Design review of the part built by this model. Coordinates are the model's own, in mm. A direction names the side the tool comes from. Round coordinates to 2 decimals unless told otherwise and drop trailing zeros. Loops run counter-clockwise (first coordinate to the right, second up) from the corner with the lowest first, then second, coordinate; pieces in that order, holes last. Notation, with made-up numbers: (8.25, 56) -> (47.25, 56) arc R6 ccw to (47.25, 63) -> close; hole circle Ø8 at (30, -37). An arc over 180 degrees is marked (long way). Answer as CSV lines item,"result". Start each with the question number.
(1) For P1, Ø1.5, axis at y = -10, z = 22, coming from the +X side; P2, Ø8.5, axis at x = -106, y = -23, coming from the +Z side; P3, Ø9.5, axis at x = -102.5, y = -17, coming from the -Z side, all flat-tipped, find the tip position at first contact; note any pin that passes through.
(2) To check wall thickness, follow line 1 (X direction, y = -15, z = 33); line 2 (Y direction, x = -36.5, z = 17); line 3 (X direction, y = -8.5, z = 16). State the ranges of each line that lie inside material, in increasing order. Write a range as from..to.
(3) Draft analysis for pull direction X (two halves, no side actions). For faces 4 (the face through (115.983, -17.769, -24.608)), 5 (the face through (-115.983, -17.769, -24.608)), 6 (the face through (114.96, -17.69, 11.75)), state which applies: +X half, -X half, draft (parallel to the pull), parting line (faces both ways), or undercut.
(4) Take a section at B-B, the plane y = -23. Write out the cut boundary in (x, z), and give its area (3 significant figures).
(5) Take a section at C-C, the plane x = 66. Write out the cut boundary in (y, z), and give its area (3 significant figures).
(6) Machinability: for faces 1 (the face through (-1, -2, 48.064)), 2 (the face through (100, -19, -33.216)), 3 (the face through (101, -19, -25.596)), which of the approach directions +Z, -Z, +X, -X, +Y, -Y give a long, thin tool a straight path to every point of the face, cutting with its end or side? Answer none if there is none.
(7) Take a section at D-D, the plane z = -22. Write out the cut boundary in (x, y), and give its area (3 significant figures).
(8) Take a section at A-A, the plane z = -8. Write out the cut boundary in (x, y), and give its area (3 significant figures).
from build123d import *

# Parameters (mm, degrees)
F0_W     = 246.3848441839
F0_H     = 96.1289182305
F1_DEPTH = 3.81
F2_R     = 14.1092662394
F3_DEPTH = 81.28
F5_DEPTH = 25.4
F6_R     = 14.1092662394
F7_DEPTH = 7.62


# Not quite as in the source:
# - a pattern or mirror of a feature is missing from the dataset's text; its kind, count and spacing are read off the source's solid
# - a feature names something its author has since deleted; it is built from what else it names


with BuildPart() as f1:
    # F0 (on Front) → F1 (new body)
    with BuildSketch(Plane.XZ):
        Rectangle(F0_W, F0_H)
    extrude(amount=F1_DEPTH)

    # F2 (on face) → F3 (join)
    with BuildSketch(Plane.XY.offset(48.0644591153)):
        with BuildLine():
            ThreePointArc((-108.1859269769, -3.81), (-109.4788428986, -32.8031453268), (-84.1323126967, -18.6671093106))
            ThreePointArc((-84.1323126967, -18.6671093106), (-86.6114524229, -9.9357548511), (-93.3090499012, -3.81))
            Line((-93.3090499012, -3.81), (-108.1859269769, -3.81))
        make_face()
        with Locations((-100.8657291532, -18.3125622571)):
            Circle(F2_R, mode=Mode.SUBTRACT)
    f3 = extrude(amount=-F3_DEPTH)

    # F3_copies: F3 across plane
    add(f3.mirror(Plane(origin=(0, 0, 0), x_dir=(0, 0, 1), z_dir=(1, 0, 0))))

    # F4 (on face) → F5 (cut)
    with BuildSketch(Plane(origin=(0, 0, 0), x_dir=(-1, 0, 0), z_dir=(0, 1, 0))):
        Polygon((-113.6597358778, -48.0644591153), (-123.1800099188, 48.0619171371), (-123.192422092, 47.8396813394), (-123.192422092, -48.0644591153), align=None)
    f5 = extrude(amount=-F5_DEPTH, mode=Mode.SUBTRACT)

    # F5_copies: F5 across plane
    add(f5.mirror(Plane(origin=(0, 0, 0), x_dir=(0, 0, -1), z_dir=(-1, 0, 0))), mode=Mode.SUBTRACT)

    # F6 (on face) → F7 (join)
    with BuildSketch(Plane(origin=(0, 0, -33.2155408847), x_dir=(1, 0, 0), z_dir=(0, 0, -1))):
        with BuildLine():
            ThreePointArc((-115.130360032, 15.9625050025), (-99.772384803, 3.8619408749), (-86.5015784629, 18.2207971811))
            ThreePointArc((-86.5015784629, 18.2207971811), (-99.772384803, 32.5796534874), (-115.130360032, 20.4790893598))
            Line((-115.130360032, 20.4790893598), (-115.130360032, 15.9625050025))
        make_face()
        with Locations((-100.8657291532, 18.3125622571)):
            Circle(F6_R, mode=Mode.SUBTRACT)
        with Locations((-100.8657291532, 18.3125622571)):
            Circle(F6_R)
    f7 = extrude(amount=-F7_DEPTH)

    # F7_copies: F7 across plane
    add(f7.mirror(Plane(origin=(0, 0, 0), x_dir=(0, 0, 1), z_dir=(1, 0, 0))))


solid = f1.part
The answers:
1,P1,"x = 115.36"
1,P2,"z = -25.6"
1,P3,"z = -33.22"
2,line 1,"-116.95..-114.58, -87.15..-84.54, 84.54..87.15, 114.58..116.95"
2,line 2,"-3.81..0"
2,line 3,"-113.89..-111, -90.73..-87.61, 87.61..90.73, 111..113.89"
3,face 4,"+X half"
3,face 5,"-X half"
3,face 6,"undercut"
4,outline,"(-116.79, -16.48) -> (-115.13, -33.22) -> (-84.71, -33.22) -> (-84.71, 48.06) -> (-87.56, 48.06) -> (-87.56, -25.6) -> (-114.17, -25.6) -> (-114.17, 48.06) -> (-116.79, 48.06) -> close; (84.71, -33.22) -> (115.13, -33.22) -> (116.79, -16.48) -> (116.79, 48.06) -> (114.17, 48.06) -> (114.17, -25.6) -> (87.56, -25.6) -> (87.56, 48.06) -> (84.71, 48.06) -> close"
4,area,"1,270 mm²"
5,outline,"(-3.81, -48.06) -> (0, -48.06) -> (0, 48.06) -> (-3.81, 48.06) -> close"
5,area,"366 mm²"
6,face 1,"+Z, +X, -X, +Y, -Y"
6,face 2,"-Z, +X, -X, -Y"
6,face 3,"+Z"
7,outline,"(-116.24, -24.67) arc R16.62 ccw (long way) to (-93.31, -3.81) -> (93.31, -3.81) arc R16.62 ccw (long way) to (116.24, -24.67) -> (116.24, -12.67) arc R16.62 ccw to (108.19, -3.81) -> (116.24, -3.81) -> (116.24, 0) -> (-116.24, 0) -> (-116.24, -3.81) -> (-108.19, -3.81) arc R16.62 ccw to (-116.24, -12.67) -> close; hole circle Ø28.22 at (-100.87, -18.31); hole circle Ø28.22 at (100.87, -18.31)"
7,area,"1,320 mm²"
8,outline,"(-117.63, -3.81) -> (-108.19, -3.81) arc R16.62 ccw (long way) to (-93.31, -3.81) -> (93.31, -3.81) arc R16.62 ccw (long way) to (108.19, -3.81) -> (117.63, -3.81) -> (117.63, 0) -> (-117.63, 0) -> close; hole circle Ø28.22 at (-100.87, -18.31); hole circle Ø28.22 at (100.87, -18.31)"
8,area,"1,340 mm²"
